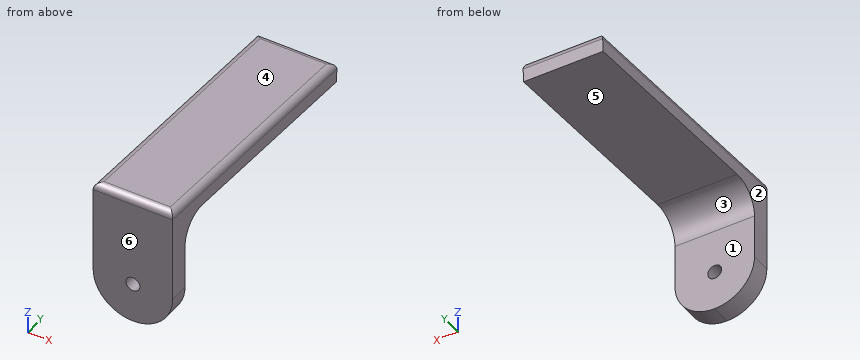
from build123d import *

# Parameters (mm, degrees)
EXTRUDE_1_DEPTH     = 12
SKETCH_2_R          = 1.05
CUT_EXTRUDE_1_DEPTH = 12
FILLET_1_R          = 1
FILLET_2_R          = 6
FILLET_3_R          = 4


with BuildPart() as part:
    # 草图1 → 凸台-拉伸1 (new body)
    with BuildSketch(Plane(origin=(0, 0, 0), x_dir=(0, 0, -1), z_dir=(1, 0, 0))):
        Polygon((2.09343825, 39.94518139), (0, 0), (20, 0), (20, 3), (3.161340376, 3), (5.089326854, 39.788173521), align=None)
    extrude(amount=EXTRUDE_1_DEPTH)

    # 草图2 → 切除-拉伸1 (cut)
    with BuildSketch(Plane(origin=(0, 3, 0), x_dir=(1, 0, 0), z_dir=(0, 1, 0))):
        with Locations(Location((6, 14, 0), (0, 0, 270))):
            Circle(SKETCH_2_R)
    extrude(amount=-CUT_EXTRUDE_1_DEPTH, mode=Mode.SUBTRACT)

    # 圆角1
    fillet_1_edges = [part.edges().sort_by_distance(p)[0] for p in [
        (6, 0, 0),
        (6, 39.94518139, -2.09343825),
        (0, 19.972590695, -1.046719125),
        (12, 19.972590695, -1.046719125),
    ]]
    fillet(fillet_1_edges, radius=FILLET_1_R)

    # 圆角2
    fillet_2_edges = [part.edges().sort_by_distance(p)[0] for p in [
        (0, 1.5, -20),
        (12, 1.5, -20),
    ]]
    fillet(fillet_2_edges, radius=FILLET_2_R - 0.0001)  # a hair under: the kernel refuses the full size

    # 圆角3
    fillet_3_edges = [part.edges().sort_by_distance(p)[0] for p in [
        (6, 3, -3.161340376),
    ]]
    fillet(fillet_3_edges, radius=FILLET_3_R)


solid = part.part
Design review of the part built by this model. Coordinates are the model's own, in mm. Face numbers are marked on the shaded views. A direction names the side the tool comes from. Give positions to 0.01 mm unless a question says otherwise; leave off trailing zeros. Loops run counter-clockwise (first coordinate to the right, second up) from the corner with the lowest first, then second, coordinate; pieces in that order, holes last. Notation, with made-up numbers: M 49,72 L 88,72 A20 cw 88,78 Z; hole C -4,30 d8. An arc over 180 degrees is marked long. One line per question, with ' | ' between items. Start each with the question number.
1. Add section B-B (z = -9.5). Write out the cut boundary in (x, y).
2. Add section C-C (x = 8.75). Write out the cut boundary in (y, z), plus the area to 3 significant figures.
3. Insertion check: P1, Ø5, axis at x = 4, z = -10, coming from the +Y side; P2, Ø8, axis at y = 7.5, z = -16.5, coming from the +X side; P3, Ø6, axis at x = 2.5, y = 10, coming from the -Z side; P4, Ø2, axis at x = 9.5, y = 9.5, coming from the +Z side. Each pin has a flat end and moves straight along its axis. Give the tip position at first contact, or say it passes through.
4. Add section A-A (x = 5.5). Write out the cut boundary in (y, z).
5. The part is to be moulded in two halves that separate along Y. For the marked faces 3, 4, 5 and 6, say which applies: released by +Y, released by -Y, zero draft, split by the parting line, or undercut.
6. For the marked faces 1 and 2, list the 3-axis set-ups (+Z, -Z, +X, -X, +Y, -Y) from which the entire face can be reached by the end or side of a thin tool; tool diameter is ignored.
7. To check wall thickness, follow L1, parallel to X at y = 1.3, z = -14; L2, parallel to Y at x = 1, z = -7.75; L3, parallel to Z at x = 7.5, y = 33. State the ranges of each line that lie inside material, in increasing order.
Worked out:
1) outline: M 0,0 L 12,0 L 12,3 L 0,3 Z
2) outline: M 0,-19.33 L 3,-19.33 L 3,-7.38 A4 cw 7.21,-3.38 L 39.79,-5.09 L 39.89,-3.09 A1 ccw 38.95,-2.04 L 1.05,-0.06 A1 ccw 0,-1.05 Z | area: 172 mm²
3) P1: stops at y = 3 | P2: passes through | P3: stops at z = -3.69 | P4: stops at z = -0.45
4) outline: M 0,-19.98 L 3,-19.98 L 3,-14.92 L 0,-14.92 Z; M 0,-13.08 L 3,-13.08 L 3,-7.38 A4 cw 7.21,-3.38 L 39.79,-5.09 L 39.89,-3.09 A1 ccw 38.95,-2.04 L 1.05,-0.06 A1 ccw 0,-1.05 Z
5) face 3: undercut | face 4: released by +Y | face 5: undercut | face 6: released by -Y
6) face 1: -Z, +X, -X, +Y | face 2: +Z, -Z, -X, +Y, -Y
7) L1: x = 0 to 4.95, 7.05 to 12 | L2: y = 0 to 3 | L3: z = -4.73 to -1.73
